The figure shows three views and two pictorial views of one solid part (mm, origin at its lowest corner). Answer the questions. Coordinates: 2 decimals unless noted, no trailing zeros. Write each loop counter-clockwise with the first axis right and the second up, starting at its lowest first coordinate (ties: lowest second). Pieces come first, ordered by that corner, then holes. Notation, with made-up numbers: (78.25, 25) - (95.25, 25) arc R18 ccw to (95.25, 47) - close; hole circle Ø5 at (1.5, 53.25). An arc over 180 degrees is marked (long way). Use a Markdown table: item, result. Add a question column.
(1) The part is cut by section C-C, the plane y = 8. Give the vertices of the cut face in (x, z).
(2) Find the intervals of material crossed by line 1 (Y direction, x = 120, z = 0.95) (1 decimal); line 2 (Y direction, x = 42, z = 1.65) (1 decimal); line 3 (X direction, y = 43, z = 1.25) (1 decimal), in increasing order. Write a range as from..to.
(3) The part is cut by section A-A, the plane z = 2.35. Give the vertices of the cut face in (x, y) (1 decimal), then the cut area to 3 significant figures.
(4) The part is cut by section B-B, the plane y = 38. Give the vertices of the cut face in (x, z), then the cut area to 3 significant figures.
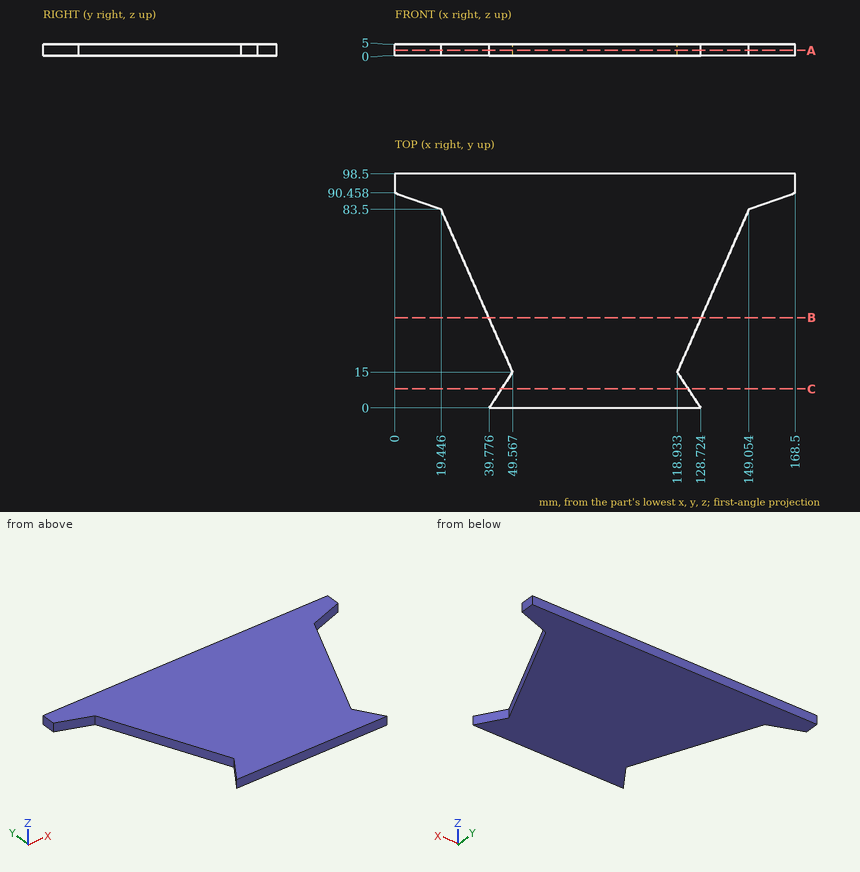
Model answer:
| question | item | result |
|---|---|---|
| 1 | outline | (45, 0) - (123.5, 0) - (123.5, 5) - (45, 5) - close |
| 2 | line 1 | 0..13.4, 17.4..98.5 |
| 2 | line 2 | 0..3.4, 32.2..98.5 |
| 2 | line 3 | 37.3..131.2 |
| 3 | outline | (0, 90.5) - (19.4, 83.5) - (49.6, 15) - (39.8, 0) - (128.7, 0) - (118.9, 15) - (149.1, 83.5) - (168.5, 90.5) - (168.5, 98.5) - (0, 98.5) - close |
| 3 | area | 10,400 mm^2 |
| 4 | outline | (39.45, 0) - (129.05, 0) - (129.05, 5) - (39.45, 5) - close |
| 4 | area | 448 mm^2 |
